```python
from build123d import *

# Parameters (mm, degrees)
BOSS_EXTRUDE1_DEPTH      = 31.22
BOSS_EXTRUDE1_DEPTH_BACK = 7
SKETCH2_R                = 6.5
SKETCH3_R                = 2.918906714
CUT_EXTRUDE1_DEPTH       = 8.36


with BuildPart() as part:
    # Sketch1 → Revolve1 (revolve)
    with BuildSketch(Plane(origin=(0, 0, 0), x_dir=(0, 0, -1), z_dir=(1, 0, 0))):
        with BuildLine():
            Line((0, 4.6), (0, -170.4))
            ThreePointArc((0, -170.4), (-1.759110094, -169.980737232), (-3.14, -168.813093167))
            Line((-3.14, -168.813093167), (-3.14, -127.813093167))
            Line((-3.14, -127.813093167), (-6.5, -88.9))
            Line((-6.5, -88.9), (-6.5, 4.6))
            Line((-6.5, 4.6), (0, 4.6))
        make_face()
    revolve(axis=Axis((0, 4.6, 0), (0, -1, 0)))

    # Sketch2 → Boss-Extrude1 (add, two sides: drawn at the far end of the back side and taken through both)
    with BuildSketch(Plane.XY.offset(-BOSS_EXTRUDE1_DEPTH_BACK)):
        Circle(SKETCH2_R)
    extrude(amount=BOSS_EXTRUDE1_DEPTH + BOSS_EXTRUDE1_DEPTH_BACK)

    # Sketch3 → Cut-Extrude1 (cut)
    with BuildSketch(Plane.XY.offset(31.22)):
        Circle(SKETCH3_R)
    extrude(amount=-CUT_EXTRUDE1_DEPTH, mode=Mode.SUBTRACT)


solid = part.part
```
Can you work these out from the model? Positions are in its coordinate system, mm. A direction names the side the tool comes from. Round coordinates to 2 decimals unless told otherwise and drop trailing zeros. Loops run counter-clockwise (first coordinate to the right, second up) from the corner with the lowest first, then second, coordinate; pieces in that order, holes last.
Item 1: Which directions (+Z, -Z, +X, -X, +Y, -Y) give clear straight access to the entire face, cutting with the end or side of a thin tool? Please do faces 5 (the flat face through (0, 0, -7)), 6 (the cylindrical face through (6.5, 2.8, -0.1)), 7 (the cylindrical face through (-2.916, 0.128, 27.099)), 8 (the cylindrical face through (-0.943, -148.026, 2.995)).
Item 2: If we mould it in two halves opening along X, with no side actions, what happens to faces 1 (the cylindrical face through (-6.5, 2.8, 0.1)), 2 (the cylindrical face through (-0.846, 6.445, 11.842)), 3 (the flat face through (0, 0, 22.86)), 4 (the flat face through (3, -1, 31.22))? For each: +X half, -X half, draft (parallel to the pull), parting line (faces both ways), or undercut.
Item 3: Please list where these lines run through material, in increasing order: L1, parallel to Y at x = 0, z = 26; L2, parallel to Y at x = 0.5, z = -3; L3, parallel to Z at x = 1.75, y = -54.
Item 4: Will these pins go through, and if not, where does the flat tip stop? pin 1 Ø3 at (y, z) = (-62.5, 4.5) entering from -X; pin 2 Ø6 at (x, z) = (4.5, 2.5) entering from +Y; pin 3 Ø4 at (x, y) = (0, -51.5) entering from -Z.
Item 5: Suppose I cut it at B-B, the plane y = -11. Write out the boundary of the cut face in (x, z).
Item 6: Suppose I cut it at A-A, the plane x = 0. Write out the boundary of the cut face in (y, z).
Reported:
1. face 5: -Z, +X, -X, +Y, -Y
1. face 6: +X, +Y
1. face 7: +Z
1. face 8: -Y
2. face 1: -X half
2. face 2: parting line
2. face 3: undercut
2. face 4: draft
3. L1: y = -6.5 to -2.92, 2.92 to 6.5
3. L2: y = -168.94 to 6.48
3. L3: z = -6.26 to 6.26
4. pin 1: stops at x = -5.77
4. pin 2: stops at y = 6.32
4. pin 3: stops at z = -6.5
5. outline: circle Ø13 at (0, 0)
6. outline: (-168.81, -3.14) - (-127.81, -3.14) - (-88.9, -6.5) - (-6.5, -6.5) - (-6.5, -7) - (6.5, -7) - (6.5, 31.22) - (2.92, 31.22) - (2.92, 22.86) - (-2.92, 22.86) - (-2.92, 31.22) - (-6.5, 31.22) - (-6.5, 6.5) - (-88.9, 6.5) - (-127.81, 3.14) - (-168.81, 3.14) arc R3.9 ccw to start
